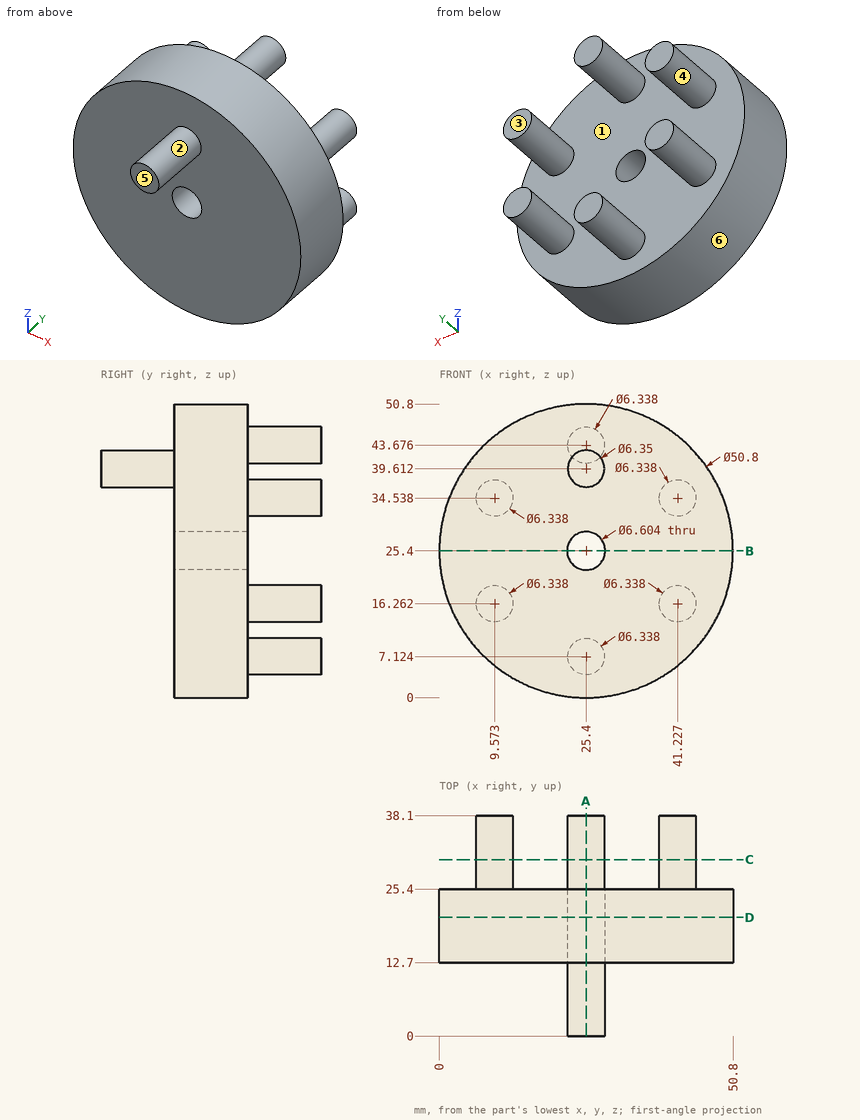
Geometry check sheet. Reference: drawing and pictorial views, mm from the part's lowest x, y, z. A direction names the side the tool comes from. Round coordinates to 2 decimals unless told otherwise and drop trailing zeros. Loops run counter-clockwise (first coordinate to the right, second up) from the corner with the lowest first, then second, coordinate; pieces in that order, holes last. Notation, with made-up numbers: (52.5, 80) - (82.5, 80) arc R34 ccw to (82.5, 112) - close; hole circle Ø11 at (53.5, 58). An arc over 180 degrees is marked (long way). Use a Markdown table: item, result.
Q1. Cross-section at A-A on x = 25.4. Record the cut outline in (y, z) (1 decimal).
Solutions:
| item | result |
|---|---|
| outline | (0, 36.4) - (12.7, 36.4) - (12.7, 28.7) - (25.4, 28.7) - (25.4, 40.5) - (38.1, 40.5) - (38.1, 46.8) - (25.4, 46.8) - (25.4, 50.8) - (12.7, 50.8) - (12.7, 42.8) - (0, 42.8) - close; (12.7, 0) - (25.4, 0) - (25.4, 4) - (38.1, 4) - (38.1, 10.3) - (25.4, 10.3) - (25.4, 22.1) - (12.7, 22.1) - close |
Q2. Cross-section at D-D on y = 20.5. Record the cut outline in (x, z), plus the area to 3 significant figures.
Solutions:
| item | result |
|---|---|
| outline | circle Ø50.8 at (25.4, 25.4); hole circle Ø6.6 at (25.4, 25.4) |
| area | 1,990 mm2 |
Q3. Material ranges on line 1 (Z direction, x = 25.4, y = 19); line 2 (Y direction, x = 35.5, z = 29.5); line 3 (Y direction, x = 12, z = 34.5), recorded low to high.
Solutions:
| item | result |
|---|---|
| line 1 | z = 0 to 22.1, 28.7 to 50.8 |
| line 2 | y = 12.7 to 25.4 |
| line 3 | y = 12.7 to 38.1 |
Q4. Draft check along X on the marked faces 4, 5 and 6. Enter one of: released by +X, released by -X, zero draft, split by the parting line, or undercut.
Solutions:
| item | result |
|---|---|
| face 4 | undercut |
| face 5 | zero draft |
| face 6 | split by the parting line |
Q5. Cross-section at C-C on y = 30.5. Record the cut outline in (x, z) (1 decimal), plus the area to 3 significant figures.
Solutions:
| item | result |
|---|---|
| outline | circle Ø6.3 at (9.6, 16.3); circle Ø6.3 at (9.6, 34.5); circle Ø6.3 at (25.4, 7.1); circle Ø6.3 at (25.4, 43.7); circle Ø6.3 at (41.2, 16.3); circle Ø6.3 at (41.2, 34.5) |
| area | 189 mm2 |
Q6. Cross-section at B-B on z = 25.4. Record the cut outline in (x, y), plus the area to 3 significant figures.
Solutions:
| item | result |
|---|---|
| outline | (0, 12.7) - (22.1, 12.7) - (22.1, 25.4) - (0, 25.4) - close; (28.7, 12.7) - (50.8, 12.7) - (50.8, 25.4) - (28.7, 25.4) - close |
| area | 561 mm2 |
Q7. Go/stop test with flat-tipped pins: P1, Ø8, axis at y = 19.5, z = 21, coming from the -X side; P2, Ø4, axis at x = 12, y = 24, coming from the +Z side; P3, Ø5.5, axis at x = 25.4, z = 25.4, coming from the -Y side (3 decimals); P4, Ø15, axis at x = 17, z = 23.5, coming from the -Y side. Record where each tip stops, or that it passes through.
Solutions:
| item | result |
|---|---|
| P1 | stops at x = 0 |
| P2 | stops at z = 48.1 |
| P3 | passes through |
| P4 | stops at y = 12.7 |
Q8. Access from +Z, -Z, +X, -X, +Y, -Y to the whole of each face (thin tool, end or side, straight path). Record for the marked faces 1, 2 and 3.
Solutions:
| item | result |
|---|---|
| face 1 | +Y |
| face 2 | -Y |
| face 3 | +Z, -Z, +X, -X, +Y |
